Autodesk Inventor part; units mm, degrees
ref_plane "YZ Plane" through (0, 0, 0) normal (1, 0, 0) x (0, 1, 0)
ref_plane "XZ Plane" through (0, 0, 0) normal (0, 1, 0) x (-1, 0, 0)
ref_plane "XY Plane" through (0, 0, 0) normal (0, 0, 1) x (1, 0, 0)
sketch "Sketch1" plane through (0, 0, 0) normal (0, 1, 0) x (-1, 0, 0)
  line L0 (0, 0) -> (-92, 0)
  line L1 (-92, 0) -> (-92, -88)
  line L2 (-92, -88) -> (0, -88)
  line L3 (0, -88) -> (0, 0)
  line L4 (0, -88) -> (-5, -88)
  line L5 (-5, -88) -> (-5, -85)
  line L6 (-5, -85) -> (0, -85)
  line L7 (0, -85) -> (0, -88)
  line L8 (0, 0) -> (-5, 0)
  line L9 (-5, 0) -> (-5, -3)
  line L10 (-5, -3) -> (0, -3)
  line L11 (0, -3) -> (0, 0)
  line L12 (-92, 0) -> (-87, 0)
  line L13 (-87, 0) -> (-87, -3)
  line L14 (-87, -3) -> (-92, -3)
  line L15 (-92, -3) -> (-92, 0)
  line L16 (-92, -88) -> (-87, -88)
  line L17 (-87, -88) -> (-87, -85)
  line L18 (-87, -85) -> (-92, -85)
  line L19 (-92, -85) -> (-92, -88)
  circle A0 centre (-9, -84) radius 1.6
  circle A1 centre (-83, -84) radius 1.6
  circle A2 centre (-9, -4) radius 1.6
  circle A3 centre (-83, -4) radius 1.6
  circle A4 centre (-46, -85) radius 1.6
  circle A5 centre (-3, -44) radius 1.6
  circle A6 centre (-89, -44) radius 1.6
  circle A7 centre (-46, -3) radius 1.6
  point P0 (0, -85)
  point P1 (0, -3)
  dimension "d6" = 82
  dimension "d8" = 88
  dimension "d10" = 92
  dimension "d11" = 5
  dimension "d12" = 3.2
  dimension "d13" = 74
  dimension "d14" = 80
  dimension "d15" = 9
  dimension "d16" = 4
  dimension "d17" = 3.2
  dimension "d18" = 46
  dimension "d19" = 44
  dimension "d20" = 3
  dimension "d21" = 3
  dimension "d22" = 3
  dimension "d23" = 3
extrude "Extrusion1" add sketch "Sketch1" along normal blind 3 contours L9 L10 L3 L6 L5 L2 L17 L18 L1 L14 L13 L0
equation "\"d15\" = -0.5 * d13 + 0.5 * d10"
equation "\"d16\" = -0.5 * d14 + 0.5 * d8"
equation "\"d18\" = 0.5 * d10"
equation "\"d19\" = 0.5 * d8"
equation "\"d21\" = d20"
equation "\"d23\" = d22"
properties part number "DummyUpperBoard"
Can you work these out from the model? Positions are in its coordinate system, mm. A direction names the side the tool comes from. Coordinates: 2 decimals unless noted, no trailing zeros. Loops run counter-clockwise (first coordinate to the right, second up) from the corner with the lowest first, then second, coordinate; pieces in that order, holes last. Notation, with made-up numbers: (49, -6.5) -> (67, -6.5) arc R18 cw to (67, 17.5) -> close; hole circle Ø1 at (14, 40). An arc over 180 degrees is marked (long way). Answer as a JSON object with one key per item and string values.
1) Imagine slicing it at A-A (x = 83). Please give me the cut outline in (y, z).
Results:
{"outline": "(0, -88) -> (3, -88) -> (3, -85.6) -> (0, -85.6) -> close; (0, -82.4) -> (3, -82.4) -> (3, -5.6) -> (0, -5.6) -> close; (0, -2.4) -> (3, -2.4) -> (3, 0) -> (0, 0) -> close"}
2) For P1, Ø1, axis at y = 1.5, z = -10, coming from the -X side; P2, Ø0.9, axis at x = 90, y = 1.5, coming from the -Z side; P3, Ø2.5, axis at x = 9, z = -4, coming from the +Y side; P4, Ø1.5, axis at x = 2, y = 2, coming from the +Z side, each with a flat end and sliding along its axis, tell me the tip position at first contact or that it passes through.
Results:
{"P1": "stops at x = 0", "P2": "stops at z = -85", "P3": "passes through", "P4": "stops at z = -3"}
3) For faces 1 (the face through (87, 1, -87)), 2 (the face through (3, 1, -3)), 3 (the face through (3, 1, -85)), 4 (the face through (47, 1, -88)), 5 (the face through (87, 1, -1)), which set-ups out of +Z, -Z, +X, -X, +Y, -Y let a thin tool reach every point of the face, with its end or its side?
Results:
{"face 1": "-Z, +X, +Y, -Y", "face 2": "+Z, -X, +Y, -Y", "face 3": "-Z, -X, +Y, -Y", "face 4": "-Z, +X, -X, +Y, -Y", "face 5": "+Z, +X, +Y, -Y"}
4) Thinking about a two-plate mould opening in Z: for faces 6 (the face through (89, 1, -3)), 7 (the face through (89, 1, -85)), 8 (the face through (81.474, 1.479, -84.481)), which applies, pulls with the +Z half, pulls with the -Z half, needs draft (parallel to the pull), parting line crosses it, or undercut?
Results:
{"face 6": "pulls with the +Z half", "face 7": "pulls with the -Z half", "face 8": "undercut"}
5) If I drill on line 1 (Z direction, x = 9, y = 1.4); line 2 (Z direction, x = 89, y = 1.35); line 3 (X direction, y = 0.9, z = -84), over which ranges is the centre line in solid material (lowest first)?
Results:
{"line 1": "z = -88 to -85.6, -82.4 to -5.6, -2.4 to 0", "line 2": "z = -85 to -45.6, -42.4 to -3", "line 3": "x = 0 to 7.4, 10.6 to 44.75, 47.25 to 81.4, 84.6 to 92"}
6) Imagine slicing it at B-B (y = 2.45). Count the separate pieces of the cut face and the enclosed holes in it, then the cut area to 3 significant figures.
Results:
{"separate pieces": "1", "enclosed holes": "8", "area": "7,970 mm^2"}
